from build123d import *

# Parameters (mm, degrees)
SKETCH1_R           = 28
SKETCH1_R_2         = 25
BOSS_EXTRUDE1_DEPTH = 15
SKETCH2_R           = 25.289752038
BOSS_EXTRUDE2_DEPTH = 1.5
FILLET1_R           = 2


with BuildPart() as part:
    # Sketch1 → Boss-Extrude1 (new body)
    with BuildSketch(Plane(origin=(0, 0, 0), x_dir=(1, 0, 0), z_dir=(0, 1, 0))):
        Circle(SKETCH1_R)
        Circle(SKETCH1_R_2, mode=Mode.SUBTRACT)
    extrude(amount=BOSS_EXTRUDE1_DEPTH)

    # Sketch2 → Boss-Extrude2 (add)
    with BuildSketch(Plane(origin=(0, 15, 0), x_dir=(1, 0, 0), z_dir=(0, 1, 0))):
        Circle(SKETCH2_R)
    extrude(amount=-BOSS_EXTRUDE2_DEPTH)

    # Fillet1
    fillet1_edges = [part.edges().sort_by_distance(p)[0] for p in [
        (-28, 15, 0),
    ]]
    fillet(fillet1_edges, radius=FILLET1_R)


solid = part.part
Read the model definition and answer for the solid it produces. Units are mm, in the model's axes. A direction names the side the tool comes from. Round coordinates to 2 decimals unless told otherwise and drop trailing zeros. Loops run counter-clockwise (first coordinate to the right, second up) from the corner with the lowest first, then second, coordinate; pieces in that order, holes last.
Q1. Section A-A on z = 0 is taken. Write down the section's boundary in (x, y).
Q2. Consider probe 1 along Z at (x, y) = (0, 4.75); probe 2 along Y at (x, z) = (10.5, 12.5). Determine where each line is inside the solid, lowest interval first.
Q3. Each of these flat-tipped pins is pushed along its axis until it touches: pin 1 (6 mm diameter, centred on y = 8, z = -8.5, fed in from -X); pin 2 (5 mm diameter, centred on x = -11.5, z = -18.5, fed in from -Y); pin 3 (3 mm diameter, centred on x = -8, y = 4, fed in from -Z). Where does it stop, or does it pass through?
Q4. Which of the six approach directions +Z, -Z, +X, -X, +Y, -Y give full straight-line access (tool end or side, diameter ignored) to faces 4 (the face through (-11, 0, -23)), 5 (the face through (23.846, 6.656, -7.509))?
Q5. Determine the mould class of faces 1 (the face through (0, 13.5, 0)), 2 (the face through (25.865, 6.409, 10.724)), 3 (the face through (0, 15, 0)) for opening direction X: released by +X, released by -X, zero draft, split by the parting line, or undercut.
Q6. Section B-B on x = 0 is taken. Write down the section's boundary in (y, z).
Output:
1. outline: (-28, 0) - (-25, 0) - (-25, 13.5) - (25, 13.5) - (25, 0) - (28, 0) - (28, 13) arc R2 ccw to (26, 15) - (-26, 15) arc R2 ccw to (-28, 13) - close
2. probe 1: z = -28 to -25, 25 to 28
2. probe 2: y = 13.5 to 15
3. pin 1: stops at x = -27.45
3. pin 2: stops at y = 13.5
3. pin 3: stops at z = -27.24
4. face 4: +Z, -Z, +X, -X, -Y
4. face 5: -Y
5. face 1: undercut
5. face 2: split by the parting line
5. face 3: zero draft
6. outline: (0, -28) - (13, -28) arc R2 ccw to (15, -26) - (15, 26) arc R2 ccw to (13, 28) - (0, 28) - (0, 25) - (13.5, 25) - (13.5, -25) - (0, -25) - close
